Answer from the drawing. Dimensions are ordinates in mm from the lowest x, y and z of the part. Round coordinates to 2 decimals unless told otherwise and drop trailing zeros. Order: outer loops, then holes, each group sorted by start corner. A loop starts at its lowest first (then second) coordinate and runs counter-clockwise, first axis right, second up. Notation, with made-up numbers: M 25,42 L 58,42 A27 cw 58,66 Z; hole C -13.75,23.5 d10. An arc over 180 degrees is marked long. Write item = value, one per line. Start each with the question number.
(1) A cutting plane is placed at A-A, the plane y = 6.5. Determine the outline of the cut face in (x, z).
(2) Each of these flat-tipped pins is pushed along its axis until it touches: pin 1 (4 mm diameter, centred on x = 78, y = 2.5, fed in from -Z); pin 2 (1.5 mm diameter, centred on y = 6, z = 36, fed in from +X); pin 3 (1.5 mm diameter, centred on y = 2.5, z = 50, fed in from +X); pin 4 (1 mm diameter, centred on y = 3.5, z = 126, fed in from +X). Where does it stop, or does it pass through?
(3) Straight lines are drawn through the part: probe 1 along Z at (x, y) = (64, 7.5); probe 2 along Z at (x, y) = (136, 3.5); probe 3 along X at (y, z) = (5.75, 147). For each, find the intervals that lie inside material, in ascending order. Write a range as from..to.
(4) A cutting plane is placed at B-B, the plane x = 69. Determine the outline of the cut face in (y, z), and give its area (3 significant figures).
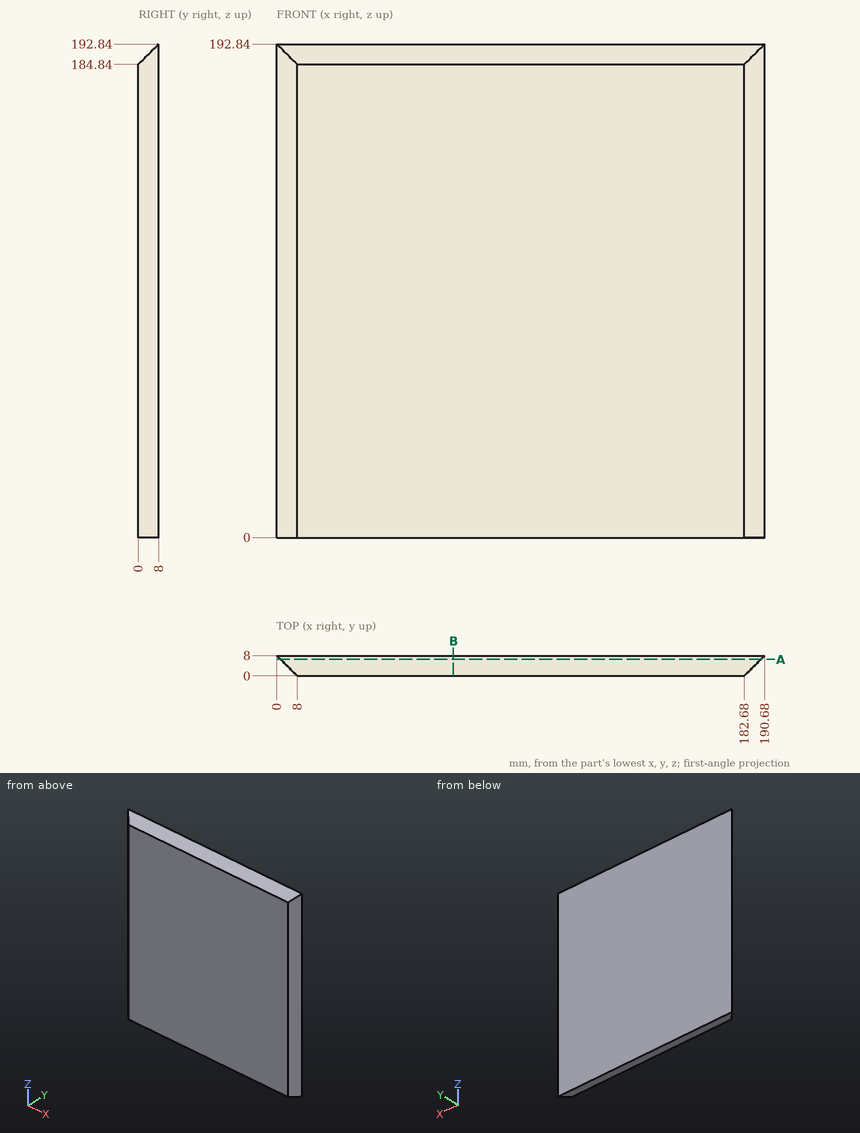
Reported:
q1.outline = M 1.5,0 L 189.18,0 L 189.18,191.34 L 1.5,191.34 Z
q2.pin_1 = 0
q2.pin_2 = 189.43
q2.pin_3 = 185.93
q2.pin_4 = 186.68
q3.probe_1 = 0..192.34
q3.probe_2 = 0..188.34
q3.probe_3 = 2.25..188.43
q4.outline = M 0,0 L 8,0 L 8,192.84 L 0,184.84 Z
q4.area = 1,510 mm²
